Can you work these out from the model? Positions are in its coordinate system, mm. A direction names the side the tool comes from. Coordinates: 2 decimals unless noted, no trailing zeros. Loops run counter-clockwise (first coordinate to the right, second up) from the corner with the lowest first, then second, coordinate; pieces in that order, holes last. Notation, with made-up numbers: (30.5, -1.75) -> (40.5, -1.75) arc R22 ccw to (40.5, 34.25) -> close; hole circle Ø4 at (15.25, 1). An arc over 180 degrees is marked (long way). Put each result on its own line as item: value. Start each with the question number.
Item 1: If we section it at A-A on z = 0: Please give me the cut outline in (x, y).
Item 2: We'd pull the mould along Z, two halves only. Please class faces 3 (the flat face through (-60, -19.05, 0)), 4 (the cylindrical face through (-55.8, 0.2, 60.8)), 5 (the cylindrical face through (0.72, -14.29, 67.51)): pulls with the +Z half, pulls with the -Z half, needs draft (parallel to the pull), parting line crosses it, or undercut.
Item 3: If we section it at B-B on x = 0: Please give me the cut outline in (y, z).
Item 4: For faces 1 (the flat face through (59.6, -9.398, -35.4)), 2 (the flat face through (-54, 19.05, 24)), which set-ups out of +Z, -Z, +X, -X, +Y, -Y let a thin tool reach every point of the face, with its end or its side?
Item 5: Will these pins go through, and if not, where does the flat tip stop? P1, Ø10, axis at y = 11, z = 59.5, coming from the +X side; P2, Ø10.5, axis at x = 69.85, z = 0, coming from the +Y side; P3, Ø2, axis at y = 13, z = -30.5, coming from the +X side; P4, Ø4, axis at y = 5.5, z = -16, coming from the +X side.
Item 6: Please list where these lines run through material, in increasing order: L1, parallel to X at y = 16, z = 15.5; L2, parallel to X at y = -17, z = 47; L3, parallel to Z at x = 60.5, y = -1. Write a range as from..to.
Item 7: If we section it at C-C on y = 0: State how many separate pieces and enclosed holes the cut face has, plus the area to 3 significant figures.
```python
from build123d import *

# Parameters (mm, degrees)
SKETCH1_W                                        = 38.1
SKETCH1_H                                        = 25.3746
CBORE_FOR_1_4_SOCKET_HEAD_CAP_SCREW1_D           = 7.1374
CBORE_FOR_1_4_SOCKET_HEAD_CAP_SCREW1_DEPTH       = 38.1
CBORE_FOR_1_4_SOCKET_HEAD_CAP_SCREW1_CBORE_D     = 11.1252
CBORE_FOR_1_4_SOCKET_HEAD_CAP_SCREW1_CBORE_DEPTH = 9.652
CBORE_FOR_1_4_SOCKET_HEAD_CAP_SCREW1_TIP         = 2.144291291
F_3_8_16_TAPPED_HOLE1_D                          = 7.9375
F_3_8_16_TAPPED_HOLE1_DEPTH                      = 38.1
F_3_8_16_TAPPED_HOLE1_TIP                        = 2.384665582
CHAMFER1_SIZE                                    = 1.524


with BuildPart() as part:
    # Sketch1 → Revolve1 (revolve)
    with BuildSketch(Plane(origin=(0, 0, 0), x_dir=(0, 1, 0), z_dir=(0, 0, 1)), mode=Mode.PRIVATE) as revolve1_sk:
        with Locations((0, 69.8373)):
            Rectangle(SKETCH1_W, SKETCH1_H)
    revolve(revolve1_sk.sketch.rotate(Axis((0, -44.45, 0), (0, 1, 0)), 270), axis=Axis((0, -44.45, 0), (0, 1, 0)))

    # CBORE for 1/4 Socket Head Cap Screw1
    with Locations(Plane(origin=(0, -19.05, 0), x_dir=(-1, 0, 0), z_dir=(0, -1, 0))):
        with Locations((0, -73.025), (-63.246, 36.5252), (63.246, 36.5252)):
            CounterBoreHole(CBORE_FOR_1_4_SOCKET_HEAD_CAP_SCREW1_D / 2, CBORE_FOR_1_4_SOCKET_HEAD_CAP_SCREW1_CBORE_D / 2, CBORE_FOR_1_4_SOCKET_HEAD_CAP_SCREW1_CBORE_DEPTH, depth=CBORE_FOR_1_4_SOCKET_HEAD_CAP_SCREW1_DEPTH)
            with Locations((0, 0, -(CBORE_FOR_1_4_SOCKET_HEAD_CAP_SCREW1_DEPTH + CBORE_FOR_1_4_SOCKET_HEAD_CAP_SCREW1_TIP / 2))):  # 118° drill point
                Cone(0, CBORE_FOR_1_4_SOCKET_HEAD_CAP_SCREW1_D / 2, CBORE_FOR_1_4_SOCKET_HEAD_CAP_SCREW1_TIP, mode=Mode.SUBTRACT)

    # 3/8-16 Tapped Hole1
    with Locations(Plane(origin=(0, -19.05, 0), x_dir=(-1, 0, 0), z_dir=(0, -1, 0))):
        with Locations((-69.85, 0)):
            Hole(F_3_8_16_TAPPED_HOLE1_D / 2, depth=F_3_8_16_TAPPED_HOLE1_DEPTH)
            with Locations((0, 0, -(F_3_8_16_TAPPED_HOLE1_DEPTH + F_3_8_16_TAPPED_HOLE1_TIP / 2))):  # 118° drill point
                Cone(0, F_3_8_16_TAPPED_HOLE1_D / 2, F_3_8_16_TAPPED_HOLE1_TIP, mode=Mode.SUBTRACT)

    # Chamfer1
    chamfer1_edges = [part.edges().sort_by_distance(p)[0] for p in [
        (0, -19.05, 57.15),
        (0, 19.05, 57.15),
        (0, 19.05, 82.5246),
        (0, -19.05, 82.5246),
    ]]
    chamfer(chamfer1_edges, length=CHAMFER1_SIZE)


solid = part.part
```
Solutions:
1. outline: (-82.52, -17.53) -> (-81, -19.05) -> (-58.67, -19.05) -> (-57.15, -17.53) -> (-57.15, 17.53) -> (-58.67, 19.05) -> (-81, 19.05) -> (-82.52, 17.53) -> close; (57.15, -17.53) -> (58.67, -19.05) -> (65.88, -19.05) -> (65.88, 19.05) -> (58.67, 19.05) -> (57.15, 17.53) -> close; (73.82, -19.05) -> (81, -19.05) -> (82.52, -17.53) -> (82.52, 17.53) -> (81, 19.05) -> (73.82, 19.05) -> close
2. face 3: needs draft
2. face 4: parting line crosses it
2. face 5: undercut
3. outline: (-19.05, -81) -> (-17.53, -82.52) -> (17.53, -82.52) -> (19.05, -81) -> (19.05, -58.67) -> (17.53, -57.15) -> (-17.53, -57.15) -> (-19.05, -58.67) -> close; (-19.05, 58.67) -> (-17.53, 57.15) -> (17.53, 57.15) -> (19.05, 58.67) -> (19.05, 69.46) -> (-9.4, 69.46) -> (-9.4, 67.46) -> (-19.05, 67.46) -> close; (-19.05, 78.59) -> (-9.4, 78.59) -> (-9.4, 76.59) -> (19.05, 76.59) -> (19.05, 81) -> (17.53, 82.52) -> (-17.53, 82.52) -> (-19.05, 81) -> close
4. face 1: -Y
4. face 2: +Z, -Z, +X, -X, +Y
5. P1: x = 61.97
5. P2: y = 19.05
5. P3: x = 77.07
5. P4: x = 81.33
6. L1: -81.06..-55.01, 55.01..81.06
6. L2: -67.83..-32.51, 32.51..67.83
6. L3: -56.13..-38.8, -34.25..56.13
7. separate pieces: 1
7. enclosed holes: 5
7. area: 11,000 mm^2
